Design review of the part shown in the three views and the two pictorial views. Dimensions are in mm from the part's minimum x, y and z. A direction names the side the tool comes from. Round coordinates to 2 decimals unless told otherwise and drop trailing zeros. Order: outer loops, then holes, each group sorted by start corner. A loop starts at its lowest first (then second) coordinate and runs counter-clockwise, first axis right, second up. Notation, with made-up numbers: M -25,45 L 8,45 A21 cw 8,83 Z; hole C -5,-29 d11. An arc over 180 degrees is marked long. Use a Markdown table: item, result. Add a question column.
(1) To check wall thickness, follow probe 1 along Z at (x, y) = (16.25, 4.5); probe 2 along X at (y, z) = (13.5, 2.25); probe 3 along Y at (x, z) = (8.5, 1.25). State the ranges of each line that lie inside material, in increasing order. Write a range as from..to.
(2) Take a section at B-B (x = 3.25). Write out the cut boundary in (y, z), then the cut area to 3 significant figures.
(3) Take a section at A-A (z = 2.75). Write out the cut boundary in (x, y), then the cut area to 3 significant figures.
(4) For pin 1 (2 mm diameter, centred on y = 14, z = 1.5, fed in from +X), flat-tipped, find the tip position at first contact; note if it passes through.
(5) Machinability: for the marked faces 1 and 2, which of the approach directions +Z, -Z, +X, -X, +Y, -Y give a long, thin tool a straight path to every point of the face, cutting with its end or side? Answer none if there is none.
(6) The part is to be moulded in two halves that separate along X. For the marked faces 3, 4 and 5, say which applies: released by +X, released by -X, zero draft, split by the parting line, or undercut.
(7) Take a section at C-C (y = 21.5). Write out the cut boundary in (x, z).
(8) Take a section at D-D (y = 7.5). Write out the cut boundary in (x, z).
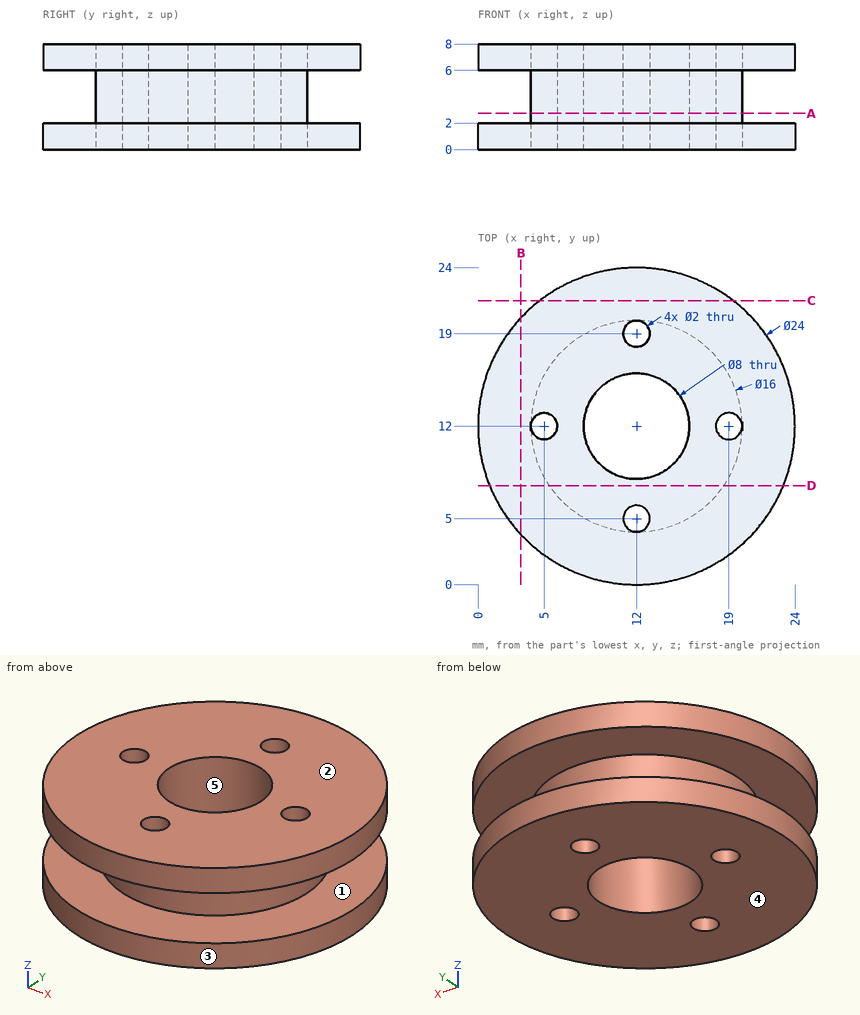
Verdict:
| question | item | result |
|---|---|---|
| 1 | probe 1 | z = 0..2, 6..8 |
| 1 | probe 2 | x = 4.14..8.29, 15.71..19.86 |
| 1 | probe 3 | y = 0.52..10.06, 13.94..23.48 |
| 2 | outline | M 3.79,0 L 20.21,0 L 20.21,2 L 3.79,2 Z; M 3.79,6 L 20.21,6 L 20.21,8 L 3.79,8 Z |
| 2 | area | 65.7 mm^2 |
| 3 | outline | C 12,12 d16; hole C 5,12 d2; hole C 12,12 d8; hole C 12,5 d2; hole C 12,19 d2; hole C 19,12 d2 |
| 3 | area | 138 mm^2 |
| 4 | pin 1 | stops at x = 23.96 |
| 5 | face 1 | none |
| 5 | face 2 | +Z, +X, -X, +Y, -Y |
| 6 | face 3 | split by the parting line |
| 6 | face 4 | zero draft |
| 6 | face 5 | undercut |
| 7 | outline | M 4.67,0 L 19.33,0 L 19.33,2 L 4.67,2 Z; M 4.67,6 L 19.33,6 L 19.33,8 L 4.67,8 Z |
| 8 | outline | M 0.88,0 L 23.12,0 L 23.12,2 L 18.61,2 L 18.61,6 L 23.12,6 L 23.12,8 L 0.88,8 L 0.88,6 L 5.39,6 L 5.39,2 L 0.88,2 Z |
